Drawing for the job (mm, zero at the part's lowest x, y, z). Round coordinates to 2 decimals unless told otherwise and drop trailing zeros. Loops run counter-clockwise (first coordinate to the right, second up) from the corner with the lowest first, then second, coordinate; pieces in that order, holes last. Notation, with made-up numbers: M 34.5,2.5 L 58.5,2.5 A18 cw 58.5,9.5 Z; hole C 23.25,-29 d1. An arc over 180 degrees is marked long. Answer in a Markdown table with one row per item.
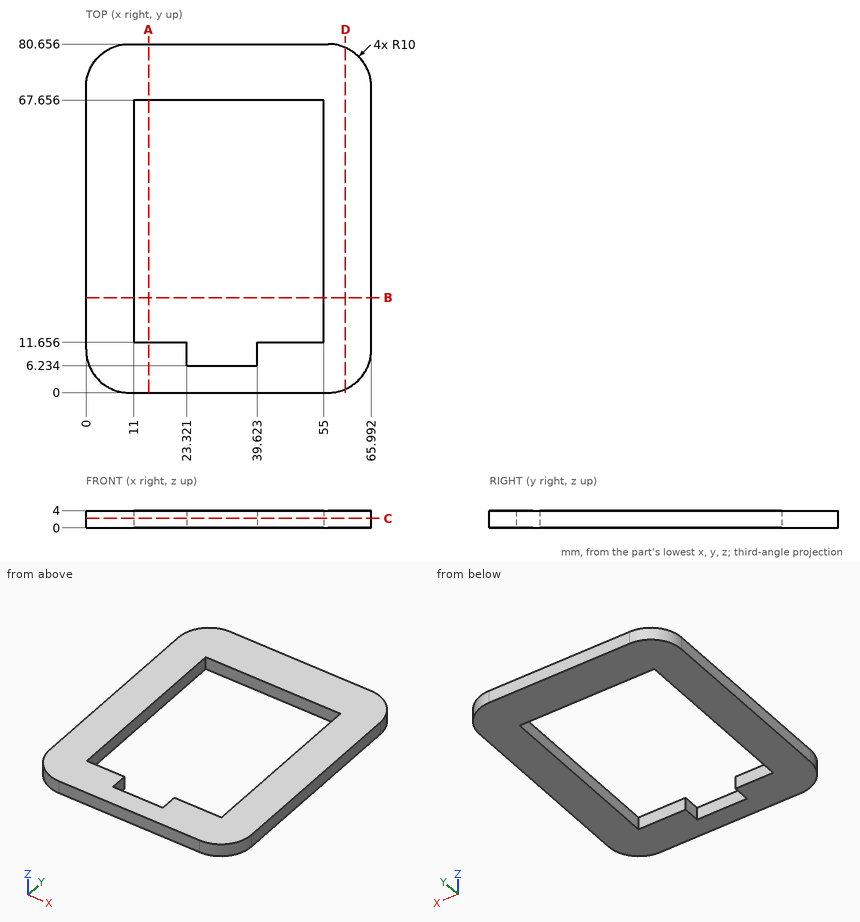
1. Saw through at A-A (x = 14.5). Write the cut outline in (y, z).
Verdict:
| item | result |
|---|---|
| outline | M 0,0 L 11.66,0 L 11.66,4 L 0,4 Z; M 67.66,0 L 80.66,0 L 80.66,4 L 67.66,4 Z |
2. Pin check, flat tip, straight feed: pin 1 (2 mm diameter, centred on x = 31, z = 2, fed in from -Y). Stop position of the tip, or through.
Verdict:
| item | result |
|---|---|
| pin 1 | stops at y = 0 |
3. Saw through at B-B (y = 22). Write the cut outline in (x, z).
Verdict:
| item | result |
|---|---|
| outline | M 0,0 L 11,0 L 11,4 L 0,4 Z; M 55,0 L 65.99,0 L 65.99,4 L 55,4 Z |
4. Saw through at D-D (x = 60). Write the cut outline in (y, z).
Verdict:
| item | result |
|---|---|
| outline | M 0.84,0 L 79.82,0 L 79.82,4 L 0.84,4 Z |
5. Saw through at C-C (z = 2.25). Write the cut outline in (x, y), and give its area (3 significant figures).
Verdict:
| item | result |
|---|---|
| outline | M 0,10 A10 ccw 10,0 L 55.99,0 A10 ccw 65.99,10 L 65.99,70.66 A10 ccw 55.99,80.66 L 10,80.66 A10 ccw 0,70.66 Z; hole M 11,11.66 L 23.32,11.66 L 23.32,6.23 L 39.62,6.23 L 39.62,11.66 L 55,11.66 L 55,67.66 L 11,67.66 Z |
| area | 2,680 mm² |
6. Wall check: probe 1 along Y at (x, z) = (24, 3.8); probe 2 along Y at (x, z) = (45, 2.55); probe 3 along X at (y, z) = (42.5, 3.35). Give the ranges that are in metal, low to high.
Verdict:
| item | result |
|---|---|
| probe 1 | y = 0 to 6.23, 67.66 to 80.66 |
| probe 2 | y = 0 to 11.66, 67.66 to 80.66 |
| probe 3 | x = 0 to 11, 55 to 65.99 |
